```python
from build123d import *

# Parameters (mm, degrees)
F0_W           = 685.8
F0_H           = 50.8
F1_DEPTH       = 19.05
F3_D           = 6.35
F3_CBORE_D     = 19.05
F3_CBORE_DEPTH = 6.35
F5_D           = 6.35
F5_CBORE_D     = 19.05
F5_CBORE_DEPTH = 6.35
F6_R           = 6.35


with BuildPart() as f1:
    # F0 (on Front) → F1 (new body)
    with BuildSketch(Plane.XZ):
        Rectangle(F0_W, F0_H)
    extrude(amount=F1_DEPTH)

    # F3 (through all)
    with Locations(Plane.XZ.offset(19.05)):
        with Locations((-317.5, 0)):
            CounterBoreHole(F3_D / 2, F3_CBORE_D / 2, F3_CBORE_DEPTH)

    # F5 (through all)
    with Locations(Plane.XZ.offset(19.05)):
        with Locations((317.5, 0), (292.1, 0), (266.7, 0), (241.3, 0), (215.9, 0), (190.5, 0), (165.1, 0), (139.7, 0), (114.3, 0), (88.9, 0)):
            CounterBoreHole(F5_D / 2, F5_CBORE_D / 2, F5_CBORE_DEPTH)

    # F6
    f6_edges = [f1.edges().sort_by_distance(p)[0] for p in [
        (0, -19.05, 25.4),
        (-342.9, -19.05, 0),
        (0, -19.05, -25.4),
        (342.9, -19.05, 0),
    ]]
    fillet(f6_edges, radius=F6_R)


solid = f1.part
```
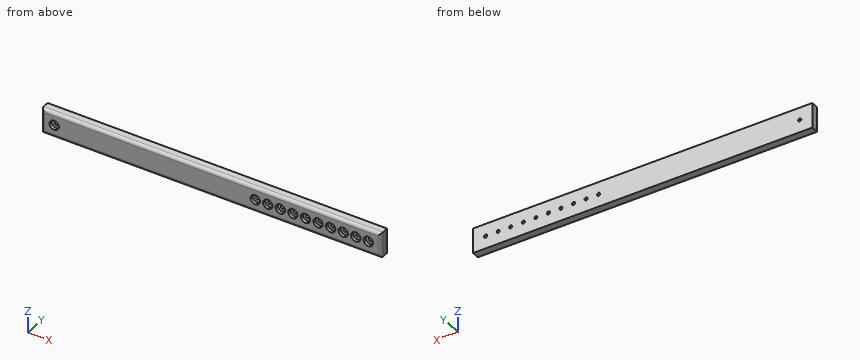
Could you check a few things on this model? Use its own coordinates, in mm. Round coordinates to 2 decimals unless told otherwise and drop trailing zeros. Loops run counter-clockwise (first coordinate to the right, second up) from the corner with the lowest first, then second, coordinate; pieces in that order, holes last. Notation, with made-up numbers: M -11,51.5 L 18,51.5 A15 cw 18,67.5 Z; hole C 52.25,4 d1. An arc over 180 degrees is marked long. Write item = value, one per line.
1. Will these pins go through, and if not, where does the flat tip stop? P1, Ø5.5, axis at x = 262.5, z = -2.5, coming from the -Y side; P2, Ø2, axis at x = 171, y = -14, coming from the -Z side.
Results below:
P1 = -12.7
P2 = -25.39
2. I need wall thicknesses on probe 1 along Z at (x, y) = (139.7, -8.25) (3 decimals); probe 2 along Z at (x, y) = (83, -18); probe 3 along X at (y, z) = (-16.75, 22). Which ranges of each line are inside material? Lowest first, please.
Results below:
probe_1 = -25.4 to -3.175, 3.175 to 25.4
probe_2 = -22.55 to -7.48, 7.48 to 22.55
probe_3 = -341.44 to 341.44
3. I want a section at A-A, the plane x = -298. Write out the boundary of the cut face in (y, z).
Results below:
outline = M -19.05,-19.05 A6.35 ccw -12.7,-25.4 L 0,-25.4 L 0,25.4 L -12.7,25.4 A6.35 ccw -19.05,19.05 Z
